Source: CAD feature listing. Evaluate the final solid. Frame: model axes, mm. A direction names the side the tool comes from. Coordinates: 2 decimals unless noted, no trailing zeros. Order: outer loops, then holes, each group sorted by start corner. A loop starts at its lowest first (then second) coordinate and runs counter-clockwise, first axis right, second up. Notation, with made-up numbers: (-21, 11) -> (-11, 11) arc R21 cw to (-11, 23) -> close; hole circle Ø8 at (50.25, 3.25). An arc over 180 degrees is marked (long way). Put each result on its own line as item: value.
from build123d import *

# Parameters (mm, degrees)
SKETCH2_W           = 10
SKETCH2_H           = 50
BOSS_EXTRUDE1_DEPTH = 10
SKETCH6_R           = 2.65
CUT_EXTRUDE3_DEPTH  = 11
SKETCH7_R           = 2.65
CUT_EXTRUDE4_DEPTH  = 11
SKETCH8_W           = 1.5
SKETCH8_H           = 21
BOSS_EXTRUDE2_DEPTH = 30


with BuildPart() as part:
    # Sketch2 → Boss-Extrude1 (new body)
    with BuildSketch(Plane.XY):
        with Locations((5, 25)):
            Rectangle(SKETCH2_W, SKETCH2_H)
    extrude(amount=BOSS_EXTRUDE1_DEPTH)

    # Sketch6 → Cut-Extrude3 (cut, through all)
    with BuildSketch(Plane.XY.offset(10)):
        with Locations((5, 27)):
            Circle(SKETCH6_R)
    extrude(amount=-CUT_EXTRUDE3_DEPTH, mode=Mode.SUBTRACT)

    # Sketch7 → Cut-Extrude4 (cut, through all)
    with BuildSketch(Plane.ZY):
        with Locations((5, 41)):
            Circle(SKETCH7_R)
        with Locations((5, 9)):
            Circle(SKETCH7_R)
    extrude(amount=-CUT_EXTRUDE4_DEPTH, mode=Mode.SUBTRACT)

    # Sketch8 → Boss-Extrude2 (add)
    with BuildSketch(Plane.ZY):
        with Locations((9.25, 26)):
            Rectangle(SKETCH8_W, SKETCH8_H)
        with Locations((0.75, 26)):
            Rectangle(SKETCH8_W, SKETCH8_H)
    extrude(amount=BOSS_EXTRUDE2_DEPTH)


solid = part.part
1. Cut plane D-D on x = -11. Output: boundary loops of the cut face in (y, z), plus the area to 3 significant figures.
Numbers:
outline: (15.5, 0) -> (36.5, 0) -> (36.5, 1.5) -> (15.5, 1.5) -> close; (15.5, 8.5) -> (36.5, 8.5) -> (36.5, 10) -> (15.5, 10) -> close
area: 63.0 mm2
2. First-contact query: pin 1 (3 mm diameter, centred on y = 41, z = 5, fed in from -X); pin 2 (5 mm diameter, centred on x = -16.5, z = 6.5, fed in from +Y); pin 3 (1.6 mm diameter, centred on x = -15, z = 0.5, fed in from -Y). Flat tips, straight axial feed; report the tip coordinate or a pass-through.
Numbers:
pin 1: passes through
pin 2: stops at y = 36.5
pin 3: stops at y = 15.5
3. Ray query, line 1 along Y through (x, z) = (4, 5); line 2 along Z through (x, y) = (-2, 26); line 3 along Y through (x, z) = (5, 5). Return the intervals inside material, ascending.
Numbers:
line 1: y = 0 to 6.35, 11.65 to 24.55, 29.45 to 38.35, 43.65 to 50
line 2: z = 0 to 1.5, 8.5 to 10
line 3: y = 0 to 6.35, 11.65 to 24.35, 29.65 to 38.35, 43.65 to 50
4. Cut plane B-B on y = 41. Output: boundary loops of the cut face in (x, z).
Numbers:
outline: (0, 0) -> (10, 0) -> (10, 2.35) -> (0, 2.35) -> close; (0, 7.65) -> (10, 7.65) -> (10, 10) -> (0, 10) -> close
5. Set-up query: faces 4 (the flat face through (-15, 26, 1.5)), 5 (the flat face through (-15, 15.5, 9)), 6 (the flat face through (-15, 36.5, 9)). Return all of +Z, -Z, +X, -X, +Y, -Y with unobstructed straight access to the full face (end or side cutting, diameter ignored); none if empty.
Numbers:
face 4: -X, +Y, -Y
face 5: +Z, -Z, -X, -Y
face 6: +Z, -Z, -X, +Y
6. Cut plane A-A on x = 5. Output: boundary loops of the cut face in (y, z), plus the area to 3 significant figures.
Numbers:
outline: (0, 0) -> (24.35, 0) -> (24.35, 10) -> (0, 10) -> close; (29.65, 0) -> (50, 0) -> (50, 10) -> (29.65, 10) -> close; hole circle Ø5.3 at (9, 5); hole circle Ø5.3 at (41, 5)
area: 403 mm2
7. Pull-direction query (Y, two-part tool) for faces 1 (the flat face through (-15, 26, 8.5)), 2 (the cylindrical face through (4.93, 6.649, 6.223)), 3 (the flat face through (5, 50, 5)); classes: pulls with the +Y half, pulls with the -Y half, needs draft (parallel to the pull), parting line crosses it, or undercut.
Numbers:
face 1: needs draft
face 2: undercut
face 3: pulls with the +Y half
8. Cut plane C-C on z = 3.25. Output: boundary loops of the cut face in (x, y).
Numbers:
outline: (0, 0) -> (10, 0) -> (10, 7.01) -> (0, 7.01) -> close; (0, 10.99) -> (10, 10.99) -> (10, 39.01) -> (0, 39.01) -> close; (0, 42.99) -> (10, 42.99) -> (10, 50) -> (0, 50) -> close; hole circle Ø5.3 at (5, 27)
